from build123d import *

# Parameters (mm, degrees)
F0_W     = 3.0607780209
F0_H     = 2.1009956449
F1_DEPTH = 5
F2_W     = 53.2925797864
F2_H     = 15.6581131741
F3_DEPTH = 2


with BuildPart() as f1:
    # F0 (on Front) → F1 (new body)
    with BuildSketch(Plane.XZ):
        with BuildLine():
            Line((-13.4510826319, 3.0807058793), (-20.9973859143, 3.0807058793))
            Line((-20.9973859143, 3.0807058793), (-26.770388545, -8.5309240967))
            Line((-26.770388545, -8.5309240967), (-26.3940021396, -8.5309240967))
            Line((-26.3940021396, -8.5309240967), (-26.3940021396, -9.6365026161))
            Line((-26.3940021396, -9.6365026161), (-21.3870331645, -9.6365026161))
            Line((-21.3870331645, -9.6365026161), (-21.3870331645, -11.8402632847))
            Line((-21.3870331645, -11.8402632847), (-24.6597826481, -11.8402632847))
            Line((-24.6597826481, -11.8402632847), (-24.6597826481, -10.3107876107))
            Line((-24.6597826481, -10.3107876107), (-26.3940021396, -10.3107876107))
            Line((-26.3940021396, -10.3107876107), (-26.3940021396, -13.2374753207))
            Line((-26.3940021396, -13.2374753207), (-20.359800871, -13.2374753207))
            ThreePointArc((-20.359800871, -13.2374753207), (-19.8294707851, -13.0178054066), (-19.609800871, -12.4874753207))
            Line((-19.609800871, -12.4874753207), (-19.609800871, -9.2809240967))
            ThreePointArc((-19.609800871, -9.2809240967), (-19.8294707851, -8.7505940108), (-20.359800871, -8.5309240967))
            Line((-20.359800871, -8.5309240967), (-19.2351932671, -8.5309240967))
            Line((-19.2351932671, -8.5309240967), (-16.9493351132, -3.8456239272))
            Line((-16.9493351132, -3.8456239272), (-13.144302211, -8.5309240967))
            Line((-13.144302211, -8.5309240967), (-14.130868949, -8.5309240967))
            Line((-14.130868949, -8.5309240967), (-14.130868949, -11.8141257167))
            Line((-14.130868949, -11.8141257167), (-17.3050090671, -11.8141257167))
            Line((-17.3050090671, -11.8141257167), (-17.3050090671, -8.5309240967))
            Line((-17.3050090671, -8.5309240967), (-19.167387858, -8.5309240967))
            Line((-19.167387858, -8.5309240967), (-19.167387858, -12.4874120876))
            ThreePointArc((-19.167387858, -12.4874120876), (-18.9477179439, -13.0177421735), (-18.417387858, -13.2374120876))
            Line((-18.417387858, -13.2374120876), (-12.2846849263, -13.2374120876))
            Line((-12.2846849263, -13.2374120876), (-12.2846849263, -8.5309240967))
            Line((-12.2846849263, -8.5309240967), (-11.065042235, -8.5309240967))
            ThreePointArc((-11.065042235, -8.5309240967), (-11.5953723208, -8.7505940108), (-11.815042235, -9.2809240967))
            Line((-11.815042235, -9.2809240967), (-11.815042235, -12.4874753207))
            ThreePointArc((-11.815042235, -12.4874753207), (-11.5953723208, -13.0178054066), (-11.065042235, -13.2374753207))
            Line((-11.065042235, -13.2374753207), (-5.1752589643, -13.2374753207))
            Line((-5.1752589643, -13.2374753207), (-5.1752589643, -11.9112924635))
            Line((-5.1752589643, -11.9112924635), (-10.0498311222, -11.9112924635))
            Line((-10.0498311222, -11.9112924635), (-10.0498311222, -9.8059958741))
            Line((-10.0498311222, -9.8059958741), (-5.1752589643, -9.8059958741))
            Line((-5.1752589643, -9.8059958741), (-5.1752589643, -8.5309240967))
            Line((-5.1752589643, -8.5309240967), (-4.6894219704, -8.5309240967))
            Line((-4.6894219704, -8.5309240967), (-4.6894219704, -13.2374753207))
            Line((-4.6894219704, -13.2374753207), (-2.891822136, -13.2374753207))
            Line((-2.891822136, -13.2374753207), (-2.891822136, -11.6197903603))
            Line((-2.891822136, -11.6197903603), (0.1689558849, -11.6197903603))
            Line((0.1689558849, -11.6197903603), (0.1689558849, -13.2374753207))
            Line((0.1689558849, -13.2374753207), (2.096112119, -13.2374753207))
            Line((2.096112119, -13.2374753207), (2.096112119, -8.5309240967))
            Line((2.096112119, -8.5309240967), (2.4571896065, -8.5309240967))
            Line((2.4571896065, -8.5309240967), (7.3034735397, -4.2975358665))
            Line((7.3034735397, -4.2975358665), (6.7291194573, -8.5309240967))
            Line((6.7291194573, -8.5309240967), (3.2661118247, -8.5309240967))
            ThreePointArc((3.2661118247, -8.5309240967), (2.7357817388, -8.7505940108), (2.5161118247, -9.2809240967))
            Line((2.5161118247, -9.2809240967), (2.5161118247, -12.4874753207))
            ThreePointArc((2.5161118247, -12.4874753207), (2.7357817388, -13.0178054066), (3.2661118247, -13.2374753207))
            Line((3.2661118247, -13.2374753207), (9.1558950953, -13.2374753207))
            Line((9.1558950953, -13.2374753207), (9.1558950953, -11.9984643534))
            Line((9.1558950953, -11.9984643534), (4.2813229375, -11.9984643534))
            Line((4.2813229375, -11.9984643534), (4.2813229375, -11.445844546))
            Line((4.2813229375, -11.445844546), (8.6850486696, -11.445844546))
            Line((8.6850486696, -11.445844546), (8.6850486696, -10.4135535657))
            Line((8.6850486696, -10.4135535657), (4.2813229375, -10.4135535657))
            Line((4.2813229375, -10.4135535657), (4.2813229375, -9.805932641))
            Line((4.2813229375, -9.805932641), (9.1558950953, -9.805932641))
            Line((9.1558950953, -9.805932641), (9.1558950953, -8.5309240967))
            Line((9.1558950953, -8.5309240967), (10.1831596047, -8.5309240967))
            ThreePointArc((10.1831596047, -8.5309240967), (9.6528295188, -8.7505940108), (9.4331596047, -9.2809240967))
            Line((9.4331596047, -9.2809240967), (9.4331596047, -10.550885953))
            ThreePointArc((9.4331596047, -10.550885953), (9.6528295188, -11.0812160389), (10.1831596047, -11.300885953))
            Line((10.1831596047, -11.300885953), (14.1622014344, -11.300885953))
            Line((14.1622014344, -11.300885953), (14.1622014344, -11.9984643534))
            Line((14.1622014344, -11.9984643534), (9.4331596047, -11.9984643534))
            Line((9.4331596047, -11.9984643534), (9.4331596047, -13.2374120876))
            Line((9.4331596047, -13.2374120876), (15.0284558833, -13.2374120876))
            ThreePointArc((15.0284558833, -13.2374120876), (15.5587859692, -13.0177421735), (15.7784558833, -12.4874120876))
            Line((15.7784558833, -12.4874120876), (15.7784558833, -11.1678693146))
            ThreePointArc((15.7784558833, -11.1678693146), (15.5587859692, -10.6375392287), (15.0284558833, -10.4178693146))
            Line((15.0284558833, -10.4178693146), (11.2140327692, -10.4178693146))
            Line((11.2140327692, -10.4178693146), (11.2140327692, -9.7743598744))
            Line((11.2140327692, -9.7743598744), (15.7784558833, -9.7743598744))
            Line((15.7784558833, -9.7743598744), (15.7784558833, -8.5309240967))
            Line((15.7784558833, -8.5309240967), (12.7156563103, -8.5309240967))
            Line((12.7156563103, -8.5309240967), (17.5534840673, -4.2975358665))
            Line((17.5534840673, -4.2975358665), (17.0895829797, -8.5309240967))
            Line((17.0895829797, -8.5309240967), (17.0398395211, -8.5309240967))
            ThreePointArc((17.0398395211, -8.5309240967), (16.5095094352, -8.7505940108), (16.2898395211, -9.2809240967))
            Line((16.2898395211, -9.2809240967), (16.2898395211, -10.550885953))
            ThreePointArc((16.2898395211, -10.550885953), (16.5095094352, -11.0812160389), (17.0398395211, -11.300885953))
            Line((17.0398395211, -11.300885953), (21.0188813508, -11.300885953))
            Line((21.0188813508, -11.300885953), (21.0188813508, -11.9984643534))
            Line((21.0188813508, -11.9984643534), (16.2898395211, -11.9984643534))
            Line((16.2898395211, -11.9984643534), (16.2898395211, -13.2374120876))
            Line((16.2898395211, -13.2374120876), (21.8851357996, -13.2374120876))
            ThreePointArc((21.8851357996, -13.2374120876), (22.4154658855, -13.0177421735), (22.6351357996, -12.4874120876))
            Line((22.6351357996, -12.4874120876), (22.6351357996, -11.1678693146))
            ThreePointArc((22.6351357996, -11.1678693146), (22.4154658855, -10.6375392287), (21.8851357996, -10.4178693146))
            Line((21.8851357996, -10.4178693146), (18.0707126856, -10.4178693146))
            Line((18.0707126856, -10.4178693146), (18.0707126856, -9.7743598744))
            Line((18.0707126856, -9.7743598744), (22.6351357996, -9.7743598744))
            Line((22.6351357996, -9.7743598744), (22.6351357996, -8.5309240967))
            Line((22.6351357996, -8.5309240967), (23.4516598284, -8.5309240967))
            Line((23.4516598284, -8.5309240967), (25.7711652666, 3.0807058793))
            Line((25.7711652666, 3.0807058793), (19.431181252, 3.0807058793))
            Line((19.431181252, 3.0807058793), (14.2619935796, -1.4036741341))
            Line((14.2619935796, -1.4036741341), (15.0130717084, 3.0807058793))
            Line((15.0130717084, 3.0807058793), (9.1148968786, 3.0807058793))
            Line((9.1148968786, 3.0807058793), (1.9796516281, -3.5022755619))
            Line((1.9796516281, -3.5022755619), (5.0060558133, 4.4282288291))
            Line((5.0060558133, 4.4282288291), (15.0130717084, 4.4282288291))
            Line((15.0130717084, 4.4282288291), (15.7288057171, 6.8140071817))
            Line((15.7288057171, 6.8140071817), (-11.583940126, 6.8140071817))
            Line((-11.583940126, 6.8140071817), (-12.7105582505, 4.4282288291))
            Line((-12.7105582505, 4.4282288291), (-2.5268180761, 4.4282288291))
            Line((-2.5268180761, 4.4282288291), (-6.9228359498, -5.4683336057))
            Line((-6.9228359498, -5.4683336057), (-10.288979272, -1.3234569953))
            Line((-10.288979272, -1.3234569953), (-4.2719710618, 3.0807058793))
            Line((-4.2719710618, 3.0807058793), (-9.4190677628, 3.0807058793))
            Line((-9.4190677628, 3.0807058793), (-15.5823286623, -1.0281349532))
            Line((-15.5823286623, -1.0281349532), (-13.4510826319, 3.0807058793))
        make_face()
        with Locations((-1.3614331256, -9.5814219192)):
            Rectangle(F0_W, F0_H, mode=Mode.SUBTRACT)
    extrude(amount=F1_DEPTH)

    # F2 (on face) → F3 (cut)
    with BuildSketch(Plane.XZ.offset(5)):
        with Locations((-0.1240986518, -0.7018675096)):
            Rectangle(F2_W, F2_H)
    extrude(amount=-F3_DEPTH, mode=Mode.SUBTRACT)


solid = f1.part
Source: CAD feature listing. Evaluate the final solid. Frame: model axes, mm. A direction names the side the tool comes from. Give positions to 0.01 mm unless a question says otherwise; leave off trailing zeros. Write each loop counter-clockwise with the first axis right and the second up, starting at its lowest first coordinate (ties: lowest second). Pieces come first, ordered by that corner, then holes. Notation, with made-up numbers: M 28,39 L 76,39 A33 ccw 76,73 Z; hole C -18.75,59 d3. An arc over 180 degrees is marked long. Return JSON: item names as keys, results as strings. Group by question number.
1) Cut plane A-A, the plane x = -0.5. Output: boundary loops of the cut face in (y, z).
2) Pull-direction query (X, two-part tool) for faces 1 (the face through (13, -2, -9.774)), 2 (the face through (-8, -4, -8.531)); classes: pulls with the +X half, pulls with the -X half, needs draft (parallel to the pull), parting line crosses it, or undercut.
3) Cut plane B-B, the plane z = 0.5. Output: boundary loops of the cut face in (x, y).
4) Material intervals for line 1 along Z through (x, y) = (8, -3.8); line 2 along Z through (x, y) = (13, -4); line 3 along Z through (x, y) = (14, -2.25), sorted ascending. Write a range as [from, to].
5) Pin query (flat end, axial travel): P1, Ø1.3, axis at y = -3.5, z = -12, coming from the -X side; P2, Ø0.6, axis at x = -11.5, y = -2, coming from the -Z side; P3, Ø1.5, axis at x = -21.5, y = -1, coming from the +Z side. Return the tip coordinate at first contact, or that it passes through.
6) Cut plane C-C, the plane y = -4.3. Give the number of separate pieces and of enclosed holes in the cut face, plus the area to 3 significant figures.
7) Set-up query: faces 3 (the face through (19, -2, -11.998)), 4 (the face through (-19.61, -2, -11)), 5 (the face through (19, -5, -11)), 6 (the face through (20, -2, -10.418)). Return all of +Z, -Z, +X, -X, +Y, -Y with unobstructed straight access to the full face (end or side cutting, diameter ignored); none if empty.
8) Cut plane D-D, the plane x = 13.5. Output: boundary loops of the cut face in (y, z).
Recorded:
{
 "1": {"outline": "M -5,-11.62 L 0,-11.62 L 0,-10.63 L -5,-10.63 Z; M -3,-8.53 L 0,-8.53 L 0,6.81 L -3,6.81 Z"},
 "2": {"face 1": "undercut", "face 2": "needs draft"},
 "3": {"outline": "M -22.28,-3 L -14.79,-3 L -14.79,0 L -22.28,0 Z; M -13.29,-3 L -7.8,-3 L -7.8,0 L -13.29,0 Z; M -4.27,-3 L 3.51,-3 L 3.51,0 L -4.27,0 Z; M 6.32,-3 L 14.58,-3 L 14.58,0 L 6.32,0 Z; M 16.46,-3 L 25.26,-3 L 25.26,0 L 16.46,0 Z"},
 "4": {"line 1": "z = [-13.24, -12], [-11.45, -10.41], [-9.81, -8.53]", "line 2": "z = [-13.24, -12], [-11.3, -10.42], [-9.77, -8.53]", "line 3": "z = [-13.24, -12], [-11.3, -10.42], [-9.77, -8.53], [-7.41, 3.08], [4.43, 6.81]"},
 "5": {"P1": "stops at x = -26.39", "P2": "stops at z = -13.23", "P3": "stops at z = 3.08"},
 "6": {"separate pieces": "7", "enclosed holes": "0", "area": "158 mm²"},
 "7": {"face 3": "+Y, -Y", "face 4": "-Z, +Y, -Y", "face 5": "+Z, -Z, +X, -X, -Y", "face 6": "+X, +Y, -Y"},
 "8": {"outline": "M -5,-13.24 L 0,-13.24 L 0,-12 L -5,-12 Z; M -5,-11.3 L 0,-11.3 L 0,-10.42 L -5,-10.42 Z; M -5,-9.77 L 0,-9.77 L 0,-8.53 L -5,-8.53 Z; M -3,-7.84 L 0,-7.84 L 0,3.08 L -3,3.08 Z; M -3,4.43 L 0,4.43 L 0,6.81 L -3,6.81 Z"}
}
